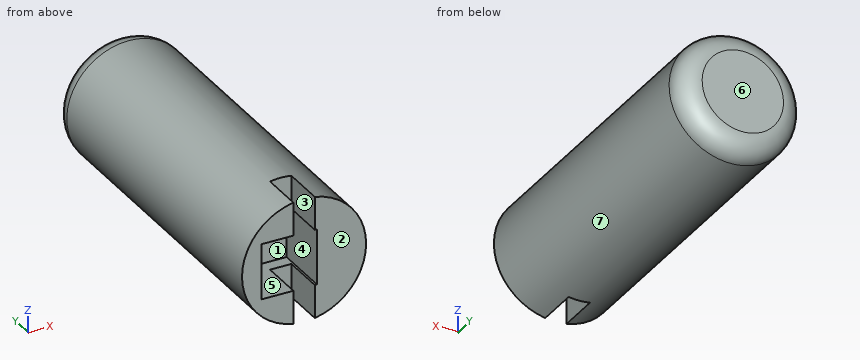
```python
from build123d import *

# Parameters (mm, degrees)
SKETCH1_R           = 2.9
BOSS_EXTRUDE1_DEPTH = 16
FILLET1_R           = 1
SKETCH2_W           = 2.6
SKETCH2_H           = 2.6
CUT_EXTRUDE1_DEPTH  = 2.6
SKETCH3_W           = 1
SKETCH3_H           = 6.114897194
CUT_EXTRUDE2_DEPTH  = 2


with BuildPart() as part:
    # Sketch1 → Boss-Extrude1 (new body)
    with BuildSketch(Plane(origin=(0, 0, 0), x_dir=(1, 0, 0), z_dir=(0, 1, 0))):
        with Locations(Location((0, 0, 0), (0, 0, 270))):
            Circle(SKETCH1_R)
    extrude(amount=BOSS_EXTRUDE1_DEPTH)

    # Fillet1
    fillet1_edges = [part.edges().sort_by_distance(p)[0] for p in [
        (0, 16, -2.9),
    ]]
    fillet(fillet1_edges, radius=FILLET1_R)

    # Sketch2 → Cut-Extrude1 (cut)
    with BuildSketch(Plane.XZ):
        with Locations((-0.7, 0)):
            Rectangle(SKETCH2_W, SKETCH2_H)
    extrude(amount=-CUT_EXTRUDE1_DEPTH, mode=Mode.SUBTRACT)

    # Sketch3 → Cut-Extrude2 (cut)
    with BuildSketch(Plane.XZ):
        Rectangle(SKETCH3_W, SKETCH3_H)
    extrude(amount=-CUT_EXTRUDE2_DEPTH, mode=Mode.SUBTRACT)


solid = part.part
```
The model under review builds one solid part; all positions refer to its coordinate system, in mm. Face numbers are marked on the shaded views. A direction names the side the tool comes from. Round coordinates to 2 decimals unless told otherwise and drop trailing zeros. Loops run counter-clockwise (first coordinate to the right, second up) from the corner with the lowest first, then second, coordinate; pieces in that order, holes last. Notation, with made-up numbers: (-11, 19.5) - (1, 19.5) arc R25 cw to (1, 50.5) - close; hole circle Ø10 at (30.5, 85.25). An arc over 180 degrees is marked (long way). Use a Markdown table: item, result. Add a question column.
Q1. For probe 1 along X at (y, z) = (11, -0.5); probe 2 along Y at (x, z) = (-0.7, 0.55); probe 3 along Z at (x, y) = (-2.05, 14.5), list the stretches that pass through material, from the lowest coordinate up.
Q2. Add section A-A (z = 0). State the section outline as (x, y) points, plus the area to 3 significant figures.
Q3. Add section B-B (x = 0). State the section outline as (y, z) points, plus the area to 3 significant figures.
Q4. Insertion check: pin 1 Ø3 at (y, z) = (10.5, -1.5) entering from +X; pin 2 Ø0.8 at (x, y) = (-1, 1) entering from -Z; pin 3 Ø0.5 at (y, z) = (1, 2.5) entering from +X; pin 4 Ø1.2 at (y, z) = (1, 1.5) entering from -X. Each pin has a flat end and moves straight along its axis. Give the tip position at first contact, or say it passes through.
Q5. Add section C-C (y = 12). State the section outline as (x, z) points, plus the area to 3 significant figures.
Q6. The part is to be moulded in two halves that separate along Z. For the marked faces 4, 5, 6 and 7, say which applies: pulls with the +Z half, pulls with the -Z half, needs draft (parallel to the pull), parting line crosses it, or undercut.
Q7. Machinability: for the marked faces 1, 2 and 3, which of the approach directions +Z, -Z, +X, -X, +Y, -Y give a long, thin tool a straight path to every point of the face, cutting with its end or side? Answer none if there is none.
Worked answers:
| question | item | result |
|---|---|---|
| 1 | probe 1 | -2.86 to 2.86 |
| 1 | probe 2 | 2.6 to 16 |
| 1 | probe 3 | -2.05 to 2.05 |
| 2 | outline | (-2.9, 0) - (-2, 0) - (-2, 2.6) - (0.6, 2.6) - (0.6, 0) - (2.9, 0) - (2.9, 15) arc R1 ccw to (1.9, 16) - (-1.9, 16) arc R1 ccw to (-2.9, 15) - close |
| 2 | area | 85.6 mm² |
| 3 | outline | (2, -2.9) - (15, -2.9) arc R1 ccw to (16, -1.9) - (16, 1.9) arc R1 ccw to (15, 2.9) - (2, 2.9) - (2, 1.3) - (2.6, 1.3) - (2.6, -1.3) - (2, -1.3) - close |
| 3 | area | 79.2 mm² |
| 4 | pin 1 | x = 2.9 |
| 4 | pin 2 | z = -2.84 |
| 4 | pin 3 | x = 1.83 |
| 4 | pin 4 | x = -2.76 |
| 5 | outline | circle Ø5.8 at (0, 0) |
| 5 | area | 26.4 mm² |
| 6 | face 4 | undercut |
| 6 | face 5 | undercut |
| 6 | face 6 | needs draft |
| 6 | face 7 | parting line crosses it |
| 7 | face 1 | -Y |
| 7 | face 2 | +Z, -Z, +X, -X, -Y |
| 7 | face 3 | +Z, -Z, -Y |
